Can you work these out from the model? Positions are in its coordinate system, mm. A direction names the side the tool comes from. Give positions to 0.01 mm unless a question says otherwise; leave off trailing zeros. Write each loop counter-clockwise with the first axis right and the second up, starting at its lowest first coordinate (ties: lowest second). Pieces come first, ordered by that corner, then holes. Notation, with made-up numbers: M 63.25,-10.5 L 92.25,-10.5 A11 cw 92.25,-4.5 Z; hole C -13.5,83.5 d11. An arc over 180 degrees is marked long. Write each question's results on one line, items separated by ' | '.
Autodesk Inventor part; units mm, degrees
ref_plane "Work Plane2" through (1183.1012, 38.0112, -55.921) normal (-0.7071, 0, -0.7071) x (0, 1, 0)
ref_plane "YZ Plane" through (0, 0, 0) normal (1, 0, 0) x (0, 1, 0)
ref_plane "XZ Plane" through (0, 0, 0) normal (0, 1, 0) x (-1, 0, 0)
sketch "Sketch1" plane through (0, 0, 0) normal (1, 0, 0) x (0, 1, 0)
  line L0 (0, 0) -> (155.1, 0)
  line L1 (155.1, 0) -> (155.1, -10)
  line L2 (0, -20) -> (0, 0)
  line L3 (155.1, -10) -> (101.6, -10)
  line L4 (101.6, -10) -> (101.6, -20)
  line L5 (101.6, -20) -> (0, -20)
  dimension "d3" = 53.5
  dimension "d4" = 155.1
  dimension "d5" = 10
  dimension "d6" = 10
  dimension "d7" = 20
  dimension "d18" = 101.6
extrude "Extrusion1" add sketch "Sketch1" along normal blind 1238.8342
chamfer "Chamfer1" distance 19.812 angle 45 1 edges at (1238.8342, 50.8, -20)
chamfer "Chamfer2" distance 19.812 angle 45 1 edges at (0, 50.8, -20)
ref_plane "Work Plane2" through (1183.1012, 38.0112, -55.921) normal (-0.7071, 0, -0.7071) x (0, 1, 0)
sketch "Sketch3" plane through (1183.1012, 38.0112, -55.921) normal (-0.7071, 0, -0.7071) x (0, 1, 0)
  line L0 (117.0888, 0) -> (14.7014, 0)
  point P0 (-38.0112, -876.121)
  dimension "d21" = 102.3874
hole "Hole1" at (1183.1012, 52.7126, -55.921) direction (0.7071, 0, 0.7071) diameter 12.7 depth 127 tip angle 118
properties part number "SkinnySideLengthPower" material "Wood (Birch)"
Item 1: If I drill on line 1 (Y direction, x = 1021, z = -14.75); line 2 (X direction, y = 128, z = -2.25); line 3 (X direction, y = 17, z = -3.5), over which ranges is the centre line in solid material (lowest first)? Write a range as from..to.
Geometry says:
line 1: y = 0..101.6 | line 2: x = 2.06..1236.77 | line 3: x = 3.31..1235.52
Item 2: For faces 1 (the face through (611, 52, -20)), 2 (the face through (611, 129, -10)), which set-ups out of +Z, -Z, +X, -X, +Y, -Y let a thin tool reach every point of the face, with its end or its side?
Geometry says:
face 1: -Z, +X, -X, +Y, -Y | face 2: -Z, +X, -X, +Y
Item 3: I'm going to push flat-ended pins straight in: pin 1 (12 mm diameter, centred on y = 76, z = -4.5, fed in from -X); pin 2 (3 mm diameter, centred on y = 60, z = -10.5, fed in from -X); pin 3 (5 mm diameter, centred on x = 584.5, z = -17.5, fed in from +Y); pin 4 (6 mm diameter, centred on x = 390.5, y = 128.5, fed in from -Z). Where does each tip first touch, or does it pass through?
Geometry says:
pin 1: stops at x = 0 | pin 2: stops at x = 8.81 | pin 3: stops at y = 101.6 | pin 4: stops at z = -10
Item 4: I want a section at B-B, the plane x = 433.5. Please give me the cut outline in (y, z), and give its area (3 significant figures).
Geometry says:
outline: M 0,-20 L 101.6,-20 L 101.6,-10 L 155.1,-10 L 155.1,0 L 0,0 Z | area: 2,570 mm2
Item 5: I want a section at A-A, the plane y = 89. Please give me the cut outline in (x, z), and give its area (3 significant figures).
Geometry says:
outline: M 0,-0.19 L 19.81,-20 L 1219.02,-20 L 1238.83,-0.19 L 1238.83,0 L 0,0 Z | area: 24,400 mm2
